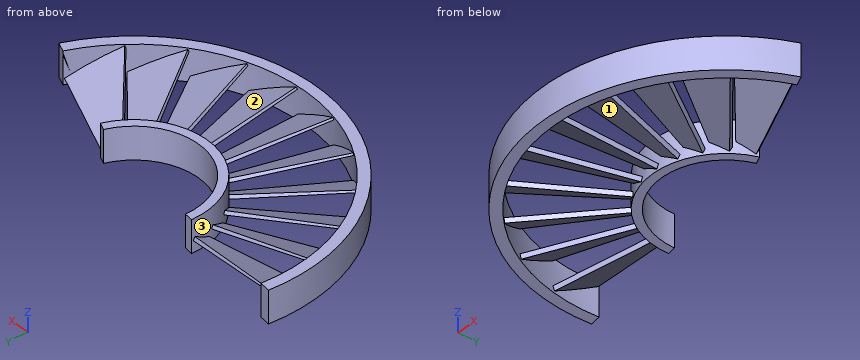
```python
from build123d import *

# Parameters (mm, degrees)
PAD036_DEPTH              = 200
TUBE014_R                 = 100
TUBE014_R_2               = 80
TUBE014_DEPTH             = 200
PAD026_DEPTH              = 100
PAD027_DEPTH              = 2
COMMON011_PLACEMENT_ANGLE = 28
ARRAY011_COUNT            = 22
ARRAY011_PLACEMENT_ANGLE  = 180
TUBE023_R                 = 85
TUBE023_R_2               = 80
TUBE023_DEPTH             = 15
TUBE024_R                 = 34
TUBE024_R_2               = 30
TUBE024_DEPTH             = 15


with BuildPart() as body037:
    # Sketch036 → Pad036 (new body)
    with BuildSketch(Plane.XY):
        Polygon((-29.110853, 1.584928), (-96.197479, 11.61747), (-96.197479, -126.516327), (86.349205, -133.978043), (86.349205, -36.423061), (25.978256, -9.215396), align=None)
    extrude(amount=PAD036_DEPTH)


with BuildPart() as tube014:
    # Tube014 → Tube014 (new body)
    with BuildSketch(Plane.XY):
        Circle(TUBE014_R)
        Circle(TUBE014_R_2, mode=Mode.SUBTRACT)
    extrude(amount=TUBE014_DEPTH)


with BuildPart() as body027:
    # Sketch026 → Pad026 (new body)
    with BuildSketch(Plane.XZ):
        Polygon((0, 0), (0, 2), (26, 0.9), (26, 0), align=None)
    extrude(amount=PAD026_DEPTH)


with BuildPart() as body027_1:
    # Body027 placement: moved
    add(body027.part.moved(Location((-5, 0, 5))))


with BuildPart() as cut003:
    # Sketch027 → Pad027 (new body)
    with BuildSketch(Plane.XY):
        Polygon((0, 0), (0, -52), (25.94305, -47.924315), (8.5, 0), align=None)
    extrude(amount=PAD027_DEPTH)


with BuildPart() as cut003_1:
    # Body028 placement: moved
    add(cut003.part.moved(Location((-5, -33, 5))))

    # Common011: intersect Body027
    add(body027_1.part, mode=Mode.INTERSECT)


with BuildPart() as cut003_2:
    # Common011 placement: moved
    add(cut003_1.part.rotate(Axis((0, 0, 0), (0, 1, 0)), COMMON011_PLACEMENT_ANGLE))

    # Array011: Cut003 ×22 about axis
    array011_axis = Axis((0, 0, 0), (0, 0, 1))


with BuildPart() as cut003_3:
    add(cut003_2.part)
    for i in range(1, ARRAY011_COUNT):
        add(cut003_2.part.rotate(array011_axis, i * 360 / ARRAY011_COUNT))


with BuildPart() as cut003_4:
    # Array011 placement: moved
    add(cut003_3.part.moved(Location((0, 0, 78))).rotate(Axis((0, 0, 78), (0, 1, 0)), ARRAY011_PLACEMENT_ANGLE))

    # Cut003: cut Tube014
    add(tube014.part, mode=Mode.SUBTRACT)


with BuildPart() as tube023:
    # Tube023 → Tube023 (new body)
    with BuildSketch(Plane.XY.offset(68.5)):
        Circle(TUBE023_R)
        Circle(TUBE023_R_2, mode=Mode.SUBTRACT)
    extrude(amount=TUBE023_DEPTH)


with BuildPart() as stator2h1:
    # Tube024 → Tube024 (new body)
    with BuildSketch(Plane.XY.offset(68.5)):
        Circle(TUBE024_R)
        Circle(TUBE024_R_2, mode=Mode.SUBTRACT)
    extrude(amount=TUBE024_DEPTH)

    # Fusion011: union Cut003, Tube023
    add(cut003_4.part)
    add(tube023.part)

    # Common019: intersect Body037
    add(body037.part, mode=Mode.INTERSECT)


solid = stator2h1.part
```
Design review of the part built by this model. Coordinates are the model's own, in mm. Face numbers are marked on the shaded views. A direction names the side the tool comes from. Give positions to 0.01 mm unless a question says otherwise; leave off trailing zeros. Order: outer loops, then holes, each group sorted by start corner. A loop starts at its lowest first (then second) coordinate and runs counter-clockwise, first axis right, second up. Notation, with made-up numbers: M 9.5,-1 L 62.5,-1 A28 ccw 62.5,18 Z; hole C 41.5,69.5 d7. An arc over 180 degrees is marked long. One line per question, with ' | ' between items. Start each with the question number.
Q1. For L1, parallel to X at y = -66, z = 73; L2, parallel to Y at x = -51.5, z = 74; L3, parallel to X at y = -4.5, z = 82.75, list the stretches that pass through material, from the lowest coordinate up. Write a range as [from, to].
Q2. For pin 1 Ø1.5 at (x, z) = (-16, 73) entering from +Y; pin 2 Ø1 at (x, y) = (33.5, -37.5) entering from -Z; pin 3 Ø2 at (x, y) = (27.5, -23.5) entering from -Z, all flat-tipped, find the tip position at first contact; note any pin that passes through.
Q3. We need section B-B (y = 4.5). Write out the cut boundary in (x, z), plus the area to 3 significant figures.
Q4. Machinability: for the marked faces 1, 2 and 3, which of the approach directions +Z, -Z, +X, -X, +Y, -Y give a long, thin tool a straight path to every point of the face, cutting with its end or side? Answer none if there is none.
Q5. We need section C-C (y = -41.5). State how many separate pieces and enclosed holes the cut face has, plus the area to 3 significant figures.
Q6. We need section A-A (x = 53). Write out the cut boundary in (y, z), plus the area to 3 significant figures.
Returned:
1) L1: [-53.56, -43.9], [-24.46, -20.68], [-4.88, -1.25], [14.29, 18.08], [36.62, 40.93], [45.21, 53.56] | L2: [-67.62, -61.22], [-40.49, -35.92], [-20.08, -16.28], [-4.25, -0.75] | L3: [-84.88, -79.87], [-33.7, -29.66]
2) pin 1: y = -24.89 | pin 2: z = 73.6 | pin 3: z = 69.47
3) outline: M -84.88,68.5 L -79.87,68.5 L -79.87,79.43 L -52.27,77.12 L -55.91,78.94 L -79.87,80.75 L -79.87,83.5 L -84.88,83.5 Z | area: 112 mm2
4) face 1: -Z | face 2: +Z | face 3: none
5) separate pieces: 8 | enclosed holes: 0 | area: 403 mm2
6) outline: M -66.45,68.5 L -59.92,68.5 L -59.92,76.35 L -44.43,69.47 L -43.19,71.24 L -59.92,77.96 L -59.92,83.5 L -66.45,83.5 Z; M -42.36,79.83 L -22.96,69.47 L -21.93,71.24 L -41.67,80.79 Z | area: 165 mm2
